```python
from build123d import *

# Parameters (mm, degrees)
SKETCH1_R           = 2.1
SKETCH1_W           = 22.5
SKETCH1_H           = 32.5
BOSS_EXTRUDE1_DEPTH = 5


with BuildPart() as part:
    # Sketch1 → Boss-Extrude1 (new body)
    # profile 1 of 5: a face of its own
    with BuildSketch(Plane.XY):
        Polygon((-18.75, 32.5), (-3.75, 32.5), (-3.75, 37.5), (-8.127501001, 37.5), (-14.372498999, 37.5), (-18.75, 37.5), align=None)
        with Locations((-11.25, 35)):
            Circle(SKETCH1_R, mode=Mode.SUBTRACT)
    # profile 2 of 5: a face of its own
    with BuildSketch(Plane.XY):
        with Locations((-11.25, 16.25)):
            Rectangle(SKETCH1_W, SKETCH1_H)
    # profile 3 of 5: a face of its own
    with BuildSketch(Plane.XY):
        Polygon((-3.75, -5), (-3.75, 0), (-18.75, 0), (-18.75, -5), (-14.372498999, -5), (-8.127501001, -5), align=None)
        with Locations((-11.25, -2.5)):
            Circle(SKETCH1_R, mode=Mode.SUBTRACT)
    # profile 4 of 5: a face of its own
    with BuildSketch(Plane.XY):
        with BuildLine():
            ThreePointArc((-14.372498999, -5), (-11.25, -6.5), (-8.127501001, -5))
            Line((-8.127501001, -5), (-14.372498999, -5))
        make_face()
    # profile 5 of 5: a face of its own
    with BuildSketch(Plane.XY):
        with BuildLine():
            ThreePointArc((-8.127501001, 37.5), (-11.25, 39), (-14.372498999, 37.5))
            Line((-14.372498999, 37.5), (-8.127501001, 37.5))
        make_face()
    extrude(amount=BOSS_EXTRUDE1_DEPTH)


solid = part.part
```
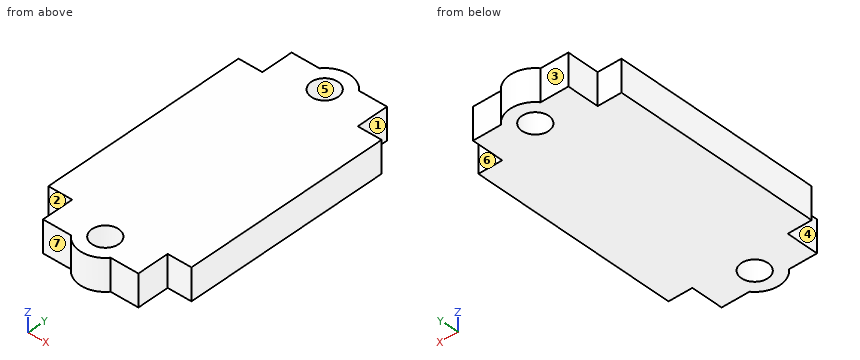
Can you work these out from the model? Positions are in its coordinate system, mm. Face numbers are marked on the shaded views. A direction names the side the tool comes from. Give positions to 0.01 mm unless a question says otherwise; leave off trailing zeros. Loops run counter-clockwise (first coordinate to the right, second up) from the corner with the lowest first, then second, coordinate; pieces in that order, holes last. Notation, with made-up numbers: M 42.25,3.25 L 81.25,3.25 A20 ccw 81.25,22.25 Z; hole C -8,-5 d8. An arc over 180 degrees is marked long. Answer in a Markdown table with one row per item.
1. If I drill on line 1 along Y through (x, z) = (-11.25, 1.6); line 2 along Y through (x, z) = (-12, 1.6); line 3 along Y through (x, z) = (-21, 3.5), over which ranges is the centre line in solid material (lowest first)?
Taken from the geometry:
| item | result |
|---|---|
| line 1 | y = -6.5 to -4.6, -0.4 to 32.9, 37.1 to 39 |
| line 2 | y = -6.43 to -4.46, -0.54 to 33.04, 36.96 to 38.93 |
| line 3 | y = 0 to 32.5 |
2. Which directions (+Z, -Z, +X, -X, +Y, -Y) give clear straight access to the entire face, cutting with the end or side of a thin tool? Please do the marked faces 1, 2 and 3.
Taken from the geometry:
| item | result |
|---|---|
| face 1 | +Z, -Z, +X, +Y |
| face 2 | +Z, -Z, -X, -Y |
| face 3 | +Z, -Z, -X, +Y |
3. Suppose I cut it at B-B on x = -11.5. Write out the boundary of the cut face in (y, z).
Taken from the geometry:
| item | result |
|---|---|
| outline | M -6.49,0 L -4.59,0 L -4.59,5 L -6.49,5 Z; M -0.41,0 L 32.91,0 L 32.91,5 L -0.41,5 Z; M 37.09,0 L 38.99,0 L 38.99,5 L 37.09,5 Z |
4. Suppose I cut it at A-A on z = 1.45. Write out the boundary of the cut face in (x, y).
Taken from the geometry:
| item | result |
|---|---|
| outline | M -22.5,0 L -18.75,0 L -18.75,-5 L -14.37,-5 A4 ccw -8.13,-5 L -3.75,-5 L -3.75,0 L 0,0 L 0,32.5 L -3.75,32.5 L -3.75,37.5 L -8.13,37.5 A4 ccw -14.37,37.5 L -18.75,37.5 L -18.75,32.5 L -22.5,32.5 Z; hole C -11.25,-2.5 d4.2; hole C -11.25,35 d4.2 |
5. For pin 1 Ø2 at (x, z) = (-6, 2) entering from -Y; pin 2 Ø1.1 at (x, z) = (-2.5, 2) entering from -Y; pin 3 Ø2.5 at (x, y) = (-11.25, 35) entering from -Z; pin 4 Ø1.1 at (x, z) = (-2, 1.5) entering from +Y, each with a flat end and sliding along its axis, tell me the tip position at first contact or that it passes through.
Taken from the geometry:
| item | result |
|---|---|
| pin 1 | stops at y = -5 |
| pin 2 | stops at y = 0 |
| pin 3 | passes through |
| pin 4 | stops at y = 32.5 |
6. Suppose I cut it at D-D on y = 36. Write out the boundary of the cut face in (x, z), plus the area to 3 significant figures.
Taken from the geometry:
| item | result |
|---|---|
| outline | M -18.75,0 L -13.1,0 L -13.1,5 L -18.75,5 Z; M -9.4,0 L -3.75,0 L -3.75,5 L -9.4,5 Z |
| area | 56.5 mm² |
7. Thinking about a two-plate mould opening in Y: for the marked faces 4, 5, 6 and 7, which applies, released by +Y, released by -Y, zero draft, split by the parting line, or undercut?
Taken from the geometry:
| item | result |
|---|---|
| face 4 | zero draft |
| face 5 | undercut |
| face 6 | released by +Y |
| face 7 | released by -Y |
8. Suppose I cut it at C-C on y = -2.5. Write out the boundary of the cut face in (x, z), plus the area to 3 significant figures.
Taken from the geometry:
| item | result |
|---|---|
| outline | M -18.75,0 L -13.35,0 L -13.35,5 L -18.75,5 Z; M -9.15,0 L -3.75,0 L -3.75,5 L -9.15,5 Z |
| area | 54.0 mm² |
